Can you work these out from the model? Positions are in its coordinate system, mm. A direction names the side the tool comes from. Round coordinates to 2 decimals unless told otherwise and drop trailing zeros. Order: outer loops, then holes, each group sorted by start corner. A loop starts at its lowest first (then second) coordinate and runs counter-clockwise, first axis right, second up. Notation, with made-up numbers: (48, 7.5) - (64, 7.5) arc R31 cw to (64, 35.5) - close; hole circle Ø7 at (45.5, -19.75). An arc over 180 degrees is marked (long way). Write item = value, one per line.
from build123d import *

# Parameters (mm, degrees)
CROQUIS3_R              = 5
SALIENTE_EXTRUIR1_DEPTH = 6
CROQUIS4_R              = 3
CORTAR_EXTRUIR1_DEPTH   = 12
CROQUIS5_R              = 5
SALIENTE_EXTRUIR2_DEPTH = 6
CROQUIS8_R              = 5
SALIENTE_EXTRUIR4_DEPTH = 6
CROQUIS9_R              = 3
CORTAR_EXTRUIR4_DEPTH   = 12
CROQUIS10_R             = 5
SALIENTE_EXTRUIR5_DEPTH = 6
CROQUIS11_R             = 3
CORTAR_EXTRUIR5_DEPTH   = 12
CORTAR_EXTRUIR7_START   = -16
CROQUIS14_R             = 3
CORTAR_EXTRUIR7_DEPTH   = 16


with BuildPart() as part:
    # Camisa → Revolución3 (revolve)
    with BuildSketch(Plane.XY):
        Polygon((-61.6, 19.5), (61.6, 19.5), (61.6, 50.1), (49.5, 50.1), (49.5, 29.193885615), (-49.5, 29.193885615), (-49.5, 50.1), (-61.6, 50.1), align=None)
        Polygon((51.5, 48.1), (59.6, 48.1), (59.6, 21.5), (-59.6, 21.5), (-59.6, 48.1), (-51.5, 48.1), (-51.5, 27.193885615), (51.5, 27.193885615), align=None, mode=Mode.SUBTRACT)
    revolve(axis=Axis((125, 0, 0), (-1, 0, 0)))

    # Croquis3 → Saliente-Extruir1 (add, symmetric)
    with BuildSketch(Plane(origin=(0, 50.1, 0), x_dir=(1, 0, 0), z_dir=(0, 1, 0))):
        with Locations(Location((-55.55, 0, 0), (0, 0, 180))):
            Circle(CROQUIS3_R)
    extrude(amount=SALIENTE_EXTRUIR1_DEPTH, both=True)

    # Croquis4 → Cortar-Extruir1 (cut)
    with BuildSketch(Plane(origin=(0, 56.1, 0), x_dir=(1, 0, 0), z_dir=(0, 1, 0))):
        with Locations(Location((-55.55, 0, 0), (0, 0, 180))):
            Circle(CROQUIS4_R)
    extrude(amount=-CORTAR_EXTRUIR1_DEPTH, mode=Mode.SUBTRACT)

    # Croquis5 → Saliente-Extruir2 (add, symmetric)
    with BuildSketch(Plane(origin=(0, 50.1, 0), x_dir=(1, 0, 0), z_dir=(0, 1, 0))):
        with Locations(Location((55.55, 0, 0), (0, 0, 180))):
            Circle(CROQUIS5_R)
    extrude(amount=SALIENTE_EXTRUIR2_DEPTH, both=True)

    # Croquis8 → Saliente-Extruir4 (add, symmetric)
    with BuildSketch(Plane(origin=(0, -50.1, 0), x_dir=(-1, 0, 0), z_dir=(0, -1, 0))):
        with Locations((55.869923699, 0)):
            Circle(CROQUIS8_R)
    extrude(amount=SALIENTE_EXTRUIR4_DEPTH, both=True)

    # Croquis9 → Cortar-Extruir4 (cut)
    with BuildSketch(Plane.XZ.offset(56.1)):
        with Locations((-55.869923699, 0)):
            Circle(CROQUIS9_R)
    extrude(amount=-CORTAR_EXTRUIR4_DEPTH, mode=Mode.SUBTRACT)

    # Croquis10 → Saliente-Extruir5 (add, symmetric)
    with BuildSketch(Plane(origin=(0, -50.1, 0), x_dir=(-1, 0, 0), z_dir=(0, -1, 0))):
        with Locations((-55.55, 0)):
            Circle(CROQUIS10_R)
    extrude(amount=SALIENTE_EXTRUIR5_DEPTH, both=True)

    # Croquis11 → Cortar-Extruir5 (cut)
    with BuildSketch(Plane.XZ.offset(56.1)):
        with Locations((55.55, 0)):
            Circle(CROQUIS11_R)
    extrude(amount=-CORTAR_EXTRUIR5_DEPTH, mode=Mode.SUBTRACT)

    # Croquis14 → Cortar-Extruir7 (cut)
    with BuildSketch(Plane(origin=(0, 56.1, 0), x_dir=(1, 0, 0), z_dir=(0, 1, 0)).offset(CORTAR_EXTRUIR7_START)):
        with Locations((55.55, 0)):
            Circle(CROQUIS14_R)
    extrude(amount=CORTAR_EXTRUIR7_DEPTH, mode=Mode.SUBTRACT)


solid = part.part
(1) Will these pins go through, and if not, where does the flat tip stop? P1, Ø2.5, axis at x = -55.5, z = -0.5, coming from the -Y side; P2, Ø9, axis at x = -55, z = -2, coming from the +Y side; P3, Ø8, axis at x = -9, z = 1.5, coming from the +Y side; P4, Ø3, axis at x = 18.5, z = -13, coming from the +Y side.
Computed:
P1 = -21.5
P2 = 56.1
P3 = 29.19
P4 = 26.83
(2) On a 3-axis mill with a long thin cutter (end or side, diameter ignored), from which of +Z, -Z, +X, -X, +Y, -Y can I reach the whole of each face in a straight line? I mean faces 1 (the face through (-53.01, -50.18, 0.9)), 2 (the face through (55.5, 46.1, 5)), 3 (the face through (-60.169, 53.019, -1.915)). Say none if no direction works.
Computed:
face_1 = -Y
face_2 = none
face_3 = +Y
(3) If we section it at B-B (z = -33): Write out the boundary of the cut face in (x, y).
Computed:
outline = (-61.6, -37.7) - (-49.5, -37.7) - (-49.5, 37.7) - (-61.6, 37.7) - close; (49.5, -37.7) - (61.6, -37.7) - (61.6, 37.7) - (49.5, 37.7) - close; hole (-59.6, -34.99) - (-51.5, -34.99) - (-51.5, 34.99) - (-59.6, 34.99) - close; hole (51.5, -34.99) - (59.6, -34.99) - (59.6, 34.99) - (51.5, 34.99) - close
(4) If I drill on line 1 (X direction, y = 35, z = 1); line 2 (Z direction, x = 21, y = 0); line 3 (Z direction, x = 42, y = 7), over which ranges is the centre line in solid material (lowest first)? Write a range as from..to.
Computed:
line_1 = -61.6..-59.6, -51.5..-49.5, 49.5..51.5, 59.6..61.6
line_2 = -29.19..-27.19, -21.5..-19.5, 19.5..21.5, 27.19..29.19
line_3 = -28.34..-26.28, -20.33..-18.2, 18.2..20.33, 26.28..28.34
(5) If we section it at C-C (x = -55.55): Write out the boundary of the cut face in (y, z), plus the area to 3 significant figures.
Computed:
outline = (-56.1, -4.99) - (-49.85, -4.99) arc R50.1 ccw to (49.85, -5) - (56.1, -5) - (56.1, -3) - (44.1, -3) - (44.1, -5) - (47.84, -5) arc R48.1 cw to (-47.84, -4.99) - (-44.1, -4.99) - (-44.1, -2.98) - (-56.1, -2.98) - close; (-56.1, 2.98) - (-44.1, 2.98) - (-44.1, 4.99) - (-47.84, 4.99) arc R48.1 cw to (47.84, 5) - (44.1, 5) - (44.1, 3) - (56.1, 3) - (56.1, 5) - (49.85, 5) arc R50.1 ccw to (-49.85, 4.99) - (-56.1, 4.99) - close; circle Ø43 at (0, 0); hole circle Ø39 at (0, 0)
area = 931 mm^2
(6) If we section it at A-A (y = 0): State how many separate pieces and enclosed holes the cut face has, plus the area to 3 significant figures.
Computed:
separate_pieces = 2
enclosed_holes = 2
area = 1,370 mm^2
(7) Thinking about a two-plate mould opening in X: for faces 4 (the face through (0.721, -27.168, -1.196)), 5 (the face through (61.6, 1, 22)), 6 (the face through (-55.8, -56.1, 3.3)), which applies, +X half, -X half, draft (parallel to the pull), parting line (faces both ways), or undercut?
Computed:
face_4 = undercut
face_5 = +X half
face_6 = draft
